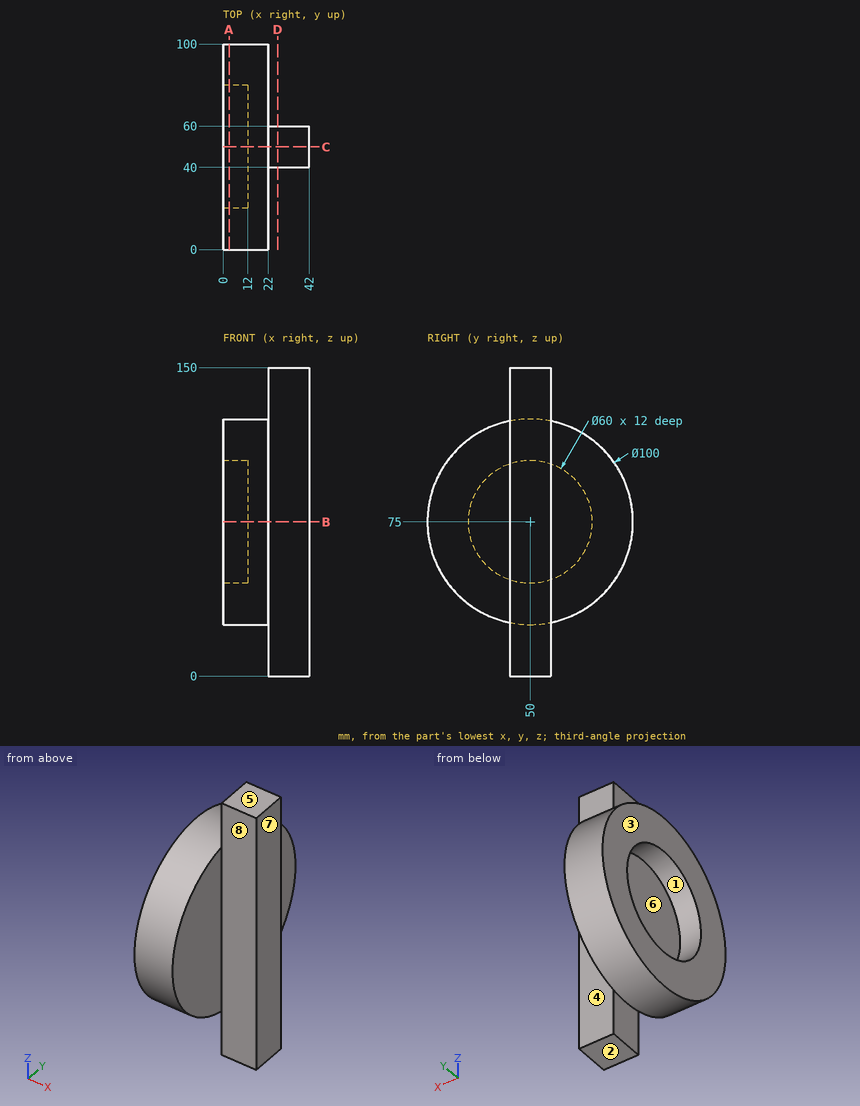
For this review, use the dimensioned drawing (mm, ordinates from the lowest corner) and the shaded views. A direction names the side the tool comes from. Round coordinates to 2 decimals unless told otherwise and drop trailing zeros. Loops run counter-clockwise (first coordinate to the right, second up) from the corner with the lowest first, then second, coordinate; pieces in that order, holes last. Notation, with made-up numbers: M 60,16 L 105,16 A21 ccw 105,36 Z; hole C -37,54.25 d10. An arc over 180 degrees is marked long. Answer as a JSON object with one key per item and string values.
(1) Tool access review of the marked faces 4, 5, 6, 7 and 8: name each direction out of +Z, -Z, +X, -X, +Y, -Y from which nothing blocks a thin tool from reaching the whole face with its end or side.
Resolved:
{"face 4": "+Z, -Z, +X, +Y", "face 5": "+Z, +X, -X, +Y, -Y", "face 6": "-X", "face 7": "+Z, -Z, +X, +Y, -Y", "face 8": "+Z, -Z, +X, -Y"}
(2) To check wall thickness, follow line 1 along Y through (x, z) = (5.5, 75); line 2 along Y through (x, z) = (30, 30); line 3 along X through (y, z) = (50.5, 142). State the ranges of each line that lie inside material, in increasing order.
Resolved:
{"line 1": "0 to 20, 80 to 100", "line 2": "40 to 60", "line 3": "22 to 42"}
(3) Clearance check with flat-ended pins moving along their axes: P1, Ø10, axis at y = 50, z = 142.5, coming from the -X side; P2, Ø8, axis at y = 21, z = 44.5, coming from the +X side; P3, Ø6, axis at x = 32, z = 72, coming from the +Y side. State where each tip first meets the part, or that it passes through.
Resolved:
{"P1": "x = 22", "P2": "x = 22", "P3": "y = 60"}
(4) Take a section at C-C on y = 50. Give the boundary of the cut face in (x, z), and give its area (3 significant figures).
Resolved:
{"outline": "M 0,25 L 22,25 L 22,0 L 42,0 L 42,150 L 22,150 L 22,125 L 0,125 L 0,105 L 12,105 L 12,45 L 0,45 Z", "area": "4,480 mm²"}
(5) Draft analysis for pull direction Z (two halves, no side actions). For the marked faces 1, 2 and 3, state which applies: released by +Z, released by -Z, zero draft, split by the parting line, or undercut.
Resolved:
{"face 1": "undercut", "face 2": "released by -Z", "face 3": "zero draft"}
(6) Take a section at A-A on x = 3. Give the boundary of the cut face in (y, z), and give its area (3 significant figures).
Resolved:
{"outline": "C 50,75 d100; hole C 50,75 d60", "area": "5,030 mm²"}
(7) Take a section at D-D on x = 26.5. Give the boundary of the cut face in (y, z).
Resolved:
{"outline": "M 40,0 L 60,0 L 60,150 L 40,150 Z"}
(8) Take a section at B-B on z = 75. Give the boundary of the cut face in (x, y).
Resolved:
{"outline": "M 0,0 L 22,0 L 22,40 L 42,40 L 42,60 L 22,60 L 22,100 L 0,100 L 0,80 L 12,80 L 12,20 L 0,20 Z"}
